Verification items for the finished model (mm, model axes). Face numbers are marked on the shaded views. A direction names the side the tool comes from. Give positions to 0.01 mm unless a question says otherwise; leave off trailing zeros. Order: outer loops, then holes, each group sorted by start corner. A loop starts at its lowest first (then second) coordinate and runs counter-clockwise, first axis right, second up. Notation, with made-up numbers: (87, -29) - (120, -29) arc R7 ccw to (120, -17) - close; hole circle Ø3 at (15, 41). An arc over 180 degrees is marked (long way). Answer as a JSON object with one key per item and string values. Group by question number.
(1) Section check B-B (z = -304). Record the boundary of the cut face in (x, y), then the cut area to 3 significant figures.
(2) Thickness scan on line 1 (X direction, y = -87.5, z = -216.5); line 2 (Z direction, x = 656.5, y = -285); line 3 (Y direction, x = 444, z = -0.5). Record the ranges inside material, lowest first.
(3) Depth check by flat-ended pin: pin 1 Ø1.5 at (x, y) = (367, -398.5) entering from +Z; pin 2 Ø4 at (y, z) = (-324, -303.5) entering from +X. Enter the tip coordinate at first touch or a pass-through.
(4) Mould release check, pull along X, two halves, no side actions. Record for the marked faces 4, 5, 6 and 7: +X half, -X half, draft (parallel to the pull), parting line (faces both ways), or undercut.
(5) Access from +Z, -Z, +X, -X, +Y, -Y to the whole of each face (thin tool, end or side, straight path). Record for the marked faces 1, 2 and 3.
(6) Section check C-C (y = -352). Record the boundary of the cut face in (x, z), then the cut area to 3 significant figures.
(7) Section check A-A (x = -383). Record the boundary of the cut face in (y, z).
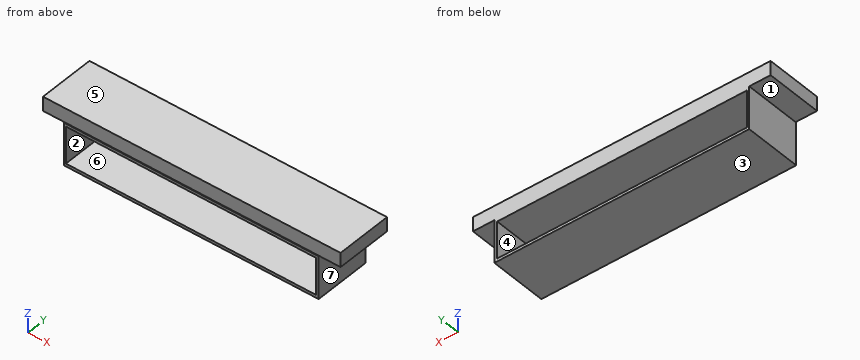
```python
from build123d import *

# Parameters (mm, degrees)
F0_W     = 20
F0_H     = 20
F0_H_2   = 260
F0_W_2   = 15
F0_W_3   = 880
F1_DEPTH = 400
F2_DEPTH = 395


# Not quite as in the source:
# - a feature names something its author has since deleted; it is built from what else it names


with BuildPart() as f1:
    # F0 (on Front) → F1 (new body)
    with BuildSketch(Plane.XZ):
        with Locations((885, -60)):
            Rectangle(F0_W, F0_H)
        Polygon((875, -70), (875, -50), (-5, -50), (-5, -70), (145, -70), align=None)
        with Locations((885, -200)):
            Rectangle(F0_W, F0_H_2)
        Polygon((-5, -70), (-5, -50), (-880, -50), (-880, -70), (-145, -70), align=None)
        with Locations((885, -340)):
            Rectangle(F0_W, F0_H)
        with Locations((-887.5, -60)):
            Rectangle(F0_W_2, F0_H)
        with Locations((435, -340)):
            Rectangle(F0_W_3, F0_H)
        with Locations((-887.5, -200)):
            Rectangle(F0_W_2, F0_H_2)
        Polygon((-5, -350), (-5, -330), (-145, -330), (-880, -330), (-880, -350), (-145, -350), align=None)
        with Locations((-887.5, -340)):
            Rectangle(F0_W_2, F0_H)
    extrude(amount=F1_DEPTH)

    # F0 (on Front) → F2 (join)
    with BuildSketch(Plane.XZ):
        Polygon((895, -50), (1045, -50), (1045, 50), (-1045, 50), (-1045, -50), (-895, -50), (-880, -50), (-5, -50), (875, -50), align=None)
    extrude(amount=F2_DEPTH)


solid = f1.part
```
Solutions:
{
 "1": {"outline": "(-895, -400) - (-880, -400) - (-880, 0) - (-895, 0) - close; (875, -400) - (895, -400) - (895, 0) - (875, 0) - close", "area": "14,000 mm2"},
 "2": {"line 1": "x = -895 to -880, 875 to 895", "line 2": "z = -350 to -330, -70 to 50", "line 3": "y = -395 to 0"},
 "3": {"pin 1": "stops at z = -50", "pin 2": "stops at x = 895"},
 "4": {"face 4": "undercut", "face 5": "draft", "face 6": "undercut", "face 7": "+X half"},
 "5": {"face 1": "-Z, -X, +Y, -Y", "face 2": "+Y, -Y", "face 3": "-Z, +X, -X, +Y, -Y"},
 "6": {"outline": "(-1045, -50) - (-895, -50) - (-895, -350) - (895, -350) - (895, -50) - (1045, -50) - (1045, 50) - (-1045, 50) - close; hole (-880, -330) - (875, -330) - (875, -70) - (-880, -70) - close", "area": "290,000 mm2"},
 "7": {"outline": "(-400, -350) - (0, -350) - (0, -330) - (-400, -330) - close; (-400, -70) - (0, -70) - (0, 50) - (-395, 50) - (-395, -50) - (-400, -50) - close"}
}
